Geometry: final body of the model. Coordinates: model frame, mm. Face numbers are marked on the shaded views. A direction names the side the tool comes from. Coordinates: 2 decimals unless noted, no trailing zeros. Loops run counter-clockwise (first coordinate to the right, second up) from the corner with the lowest first, then second, coordinate; pieces in that order, holes last. Notation, with made-up numbers: (-18.75, 42) - (35.25, 42) arc R21 ccw to (35.25, 62) - close; hole circle Ø7 at (46.25, 1.5). An arc over 180 degrees is marked (long way). Return JSON: item names as keys, results as strings.
from build123d import *

# Parameters (mm, degrees)
SKETCH_W        = 30
SKETCH_H        = 42
PAD_DEPTH       = 54
POCKET_DEPTH    = 42.001
POCKET001_DEPTH = 30.001
POCKET002_DEPTH = 42.001
POCKET003_DEPTH = 40.5
SKETCH005_W     = 12.884712
SKETCH005_H     = 5
PAD001_DEPTH    = 6
SKETCH006_W     = 8
SKETCH006_H     = 5
PAD002_DEPTH    = 5.5
SKETCH007_W     = 9
SKETCH007_H     = 5
PAD003_DEPTH    = 14
SKETCH009_R     = 1.75
POCKET004_DEPTH = 6
SKETCH010_W     = 16.115288
SKETCH010_H     = 23
PAD004_DEPTH    = 1
SKETCH011_W     = 16.658894
SKETCH011_H     = 16.071619
PAD005_DEPTH    = 1
PAD006_DEPTH    = 1
SKETCH015_R     = 1.125
POCKET005_DEPTH = 54.001
CHAMFER_SIZE    = 1.4
FILLET_R        = 0.5
SKETCH014_W     = 37.032941
SKETCH014_H     = 8.623624
POCKET006_DEPTH = 5
POCKET007_DEPTH = 47.501
FILLET001_R     = 2
FILLET002_R     = 1
FILLET003_R     = 1
FILLET004_R     = 1
FILLET005_R     = 1


with BuildPart() as part:
    # Sketch → Pad (new body)
    with BuildSketch(Plane.XY):
        with Locations((-28, -29)):
            Rectangle(SKETCH_W, SKETCH_H)
    extrude(amount=-PAD_DEPTH)

    # Sketch001 (on Face3 of Pad) → Pocket (cut, through all)
    with BuildSketch(Plane.XZ.offset(50)):
        with BuildLine():
            ThreePointArc((-43, -17.3161363132), (-32.0308923047, -38.9545248813), (-13, -54))
            Line((-13, -54), (-82.3272746231, -71.6955218441))
            Line((-82.3272746231, -71.6955218441), (-43, -17.3161363132))
        make_face()
    extrude(amount=-POCKET_DEPTH, mode=Mode.SUBTRACT)

    # Sketch002 (on Face3 of Pocket) → Pocket001 (cut, through all)
    with BuildSketch(Plane.YZ.offset(-13)):
        Polygon((0, 10), (-23, -65), (20.1488759761, -57.2462846327), align=None)
    extrude(amount=-POCKET001_DEPTH, mode=Mode.SUBTRACT)

    # Sketch004 (on Face6 of Pocket001) → Pocket002 (cut, through all)
    with BuildSketch(Plane.XZ.offset(50)):
        with BuildLine():
            ThreePointArc((-26, 0), (-13.3232341465, -48.8680892812), (21.51, -85.4117117262))
            Line((21.51, -85.4117117262), (74.53, 0))
            Line((-26, 0), (74.53, 0))
        make_face()
    extrude(amount=-POCKET002_DEPTH, mode=Mode.SUBTRACT)

    # Sketch003 (on Face1 of Pocket002) → Pocket003 (cut)
    with BuildSketch(Plane(origin=(0, -8, 0), x_dir=(-1, 0, 0), z_dir=(0, 1, 0))):
        with BuildLine():
            Line((42, 3), (42, -15))
            ThreePointArc((12.43, -53.2689919013), (31.9114915655, -37.7634197527), (42, -15))
            Line((12.43, -52.0274321222), (12.43, -53.2689919013))
            ThreePointArc((12.43, -52.0274321222), (23.2887545115, -27.0145266164), (27, 0))
            Line((27, 3), (27, 0))
            Line((42, 3), (27, 3))
        make_face()
    extrude(amount=-POCKET003_DEPTH, mode=Mode.SUBTRACT)

    # Sketch005 (on Face1 of Pocket003) → Pad001 (join)
    with BuildSketch(Plane(origin=(0, -8, 0), x_dir=(-1, 0, 0), z_dir=(0, 1, 0))):
        with Locations((20.442356, -2.5)):
            Rectangle(SKETCH005_W, SKETCH005_H)
    extrude(amount=-PAD001_DEPTH)

    # Sketch006 (on Face12 of Pad001) → Pad002 (join)
    with BuildSketch(Plane(origin=(0, -8, 0), x_dir=(-1, 0, 0), z_dir=(0, 1, 0))):
        with Locations((18, -2.5)):
            Rectangle(SKETCH006_W, SKETCH006_H)
    extrude(amount=PAD002_DEPTH)

    # Sketch007 (on Face11 of Pad002) → Pad003 (join)
    with BuildSketch(Plane.XZ.offset(50)):
        with Locations((-22.5, -2.5)):
            Rectangle(SKETCH007_W, SKETCH007_H)
    extrude(amount=-PAD003_DEPTH)

    # Sketch009 (on Face25 of Pad003) → Pocket004 (cut)
    with BuildSketch(Plane.XY):
        with Locations((-18, -6)):
            Circle(SKETCH009_R)
        with Locations((-22, -40)):
            Circle(SKETCH009_R)
    extrude(amount=-POCKET004_DEPTH, mode=Mode.SUBTRACT)

    # Sketch010 (on Face27 of Pocket004) → Pad004 (join)
    with BuildSketch(Plane.XY):
        with Locations((-34.942356, -38.5)):
            Rectangle(SKETCH010_W, SKETCH010_H)
    extrude(amount=-PAD004_DEPTH)

    # Sketch011 (on Face49 of Pad004) → Pad005 (join)
    with BuildSketch(Plane(origin=(0, -8, 0), x_dir=(-1, 0, 0), z_dir=(0, 1, 0))):
        with Locations((33.892149, -8.0883895)):
            Rectangle(SKETCH011_W, SKETCH011_H)
    extrude(amount=-PAD005_DEPTH)

    # Sketch013 (on Face47 of Pad005) → Pad006 (join)
    with BuildSketch(Plane(origin=(0, -2.8030549236, 0.8596035099), x_dir=(-1, 0, 0), z_dir=(0, 0.9560542082, -0.2931899572))):
        with BuildLine():
            Line((42.333473, -17.6579), (25.319201, -17.6579))
            ThreePointArc((13, -54.3247056888), (20.7764339487, -36.5345215912), (25.319201, -17.6579))
            Line((13, -54.3247056888), (13, -56.3377401542))
            ThreePointArc((13, -56.3377401542), (32.3236400181, -40.5294570505), (42.333473, -17.6579))
        make_face()
    extrude(amount=-PAD006_DEPTH)

    # Sketch015 (on Face37 of Pad006) → Pocket005 (cut, through all)
    with BuildSketch(Plane.XY):
        with Locations((-22, -40)):
            Circle(SKETCH015_R)
    extrude(amount=-POCKET005_DEPTH, mode=Mode.SUBTRACT)

    # Chamfer
    chamfer_edges = [part.edges().sort_by_distance(p)[0] for p in [
        (-13, -34.138239, -51.07776),
    ]]
    chamfer(chamfer_edges, length=CHAMFER_SIZE)

    # Fillet
    fillet_edges = [part.edges().sort_by_distance(p)[0] for p in [
        (-13.705397, -33.952813, -49.868456),
    ]]
    fillet(fillet_edges, radius=FILLET_R)

    # Sketch014 → Pocket006 (cut)
    with BuildSketch(Plane.YZ.offset(-13)):
        with Locations((-34.3443045, -56.822496)):
            Rectangle(SKETCH014_W, SKETCH014_H)
    extrude(amount=-POCKET006_DEPTH, mode=Mode.SUBTRACT)

    # Sketch017 (on Face39 of Pocket006) → Pocket007 (cut, through all)
    with BuildSketch(Plane.XZ.offset(50)):
        Polygon((-11.053677, -46.02187), (-17.304024, -54.523899), (-5.308009, -55.921494), align=None)
    extrude(amount=-POCKET007_DEPTH, mode=Mode.SUBTRACT)

    # Fillet001
    fillet001_edges = [part.edges().sort_by_distance(p)[0] for p in [
        (-18, -36, -2.5),
        (-22, -2.5, -2.5),
        (-14, -2.5, -2.5),
        (-14, -14, -2.5),
        (-18, -50, -2.5),
    ]]
    fillet(fillet001_edges, radius=FILLET001_R)

    # Fillet002
    fillet002_edges = [part.edges().sort_by_distance(p)[0] for p in [
        (-33.031819, -50, -37.694402),
    ]]
    fillet(fillet002_edges, radius=FILLET002_R)

    # Fillet003
    fillet003_edges = [part.edges().sort_by_distance(p)[0] for p in [
        (-22.099555, -50, -27.73103),
    ]]
    fillet(fillet003_edges, radius=FILLET003_R)

    # Fillet004
    fillet004_edges = [part.edges().sort_by_distance(p)[0] for p in [
        (-22.999305, -48.5, -28.027565),
    ]]
    fillet(fillet004_edges, radius=FILLET004_R)

    # Fillet005
    fillet005_edges = [part.edges().sort_by_distance(p)[0] for p in [
        (-32.8795, -48.5, -36.469763),
    ]]
    fillet(fillet005_edges, radius=FILLET005_R)


solid = part.part
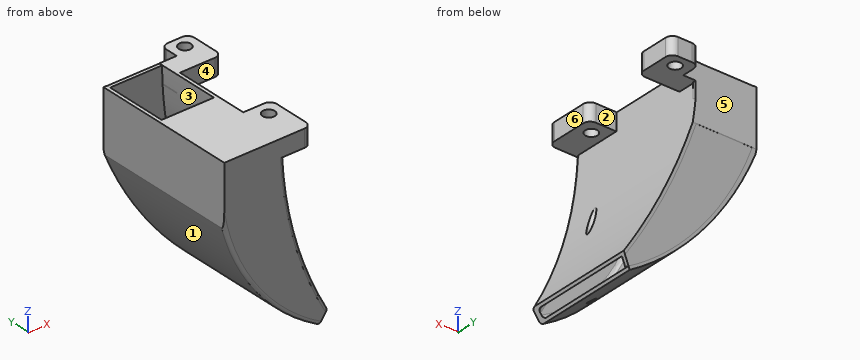
Item 1: Section query A-A, the plane y = -6. Return loops of the section in (x, z).
Worked out:
{"outline": "(-22, -5) - (-19.75, -5) - (-19.75, 0) - (-22, 0) - close; (-16.25, -5) - (-14, -5) - (-14, 0) - (-16.25, 0) - close"}
Item 2: First-contact query: pin 1 Ø3.5 at (x, y) = (-22, -40) entering from -Z; pin 2 Ø2 at (y, z) = (-39.5, -44.5) entering from +X; pin 3 Ø4 at (x, z) = (-19.5, -2.5) entering from -Y; pin 4 Ø1.5 at (y, z) = (-45, -3.5) entering from +X. Flat tips, straight axial feed; report the tip coordinate or a pass-through.
Worked out:
{"pin 1": "z = -49.78", "pin 2": "x = -15.11", "pin 3": "y = -50", "pin 4": "x = -18"}
Item 3: Ray query, probe 1 along Y at (x, z) = (-30.5, -6.5); probe 2 along Y at (x, z) = (-22, -31) (3 decimals); probe 3 along Z at (x, y) = (-38, -45). Return the intervals inside material, ascending. Write a range as from..to.
Worked out:
{"probe 1": "-50..-48.5, -9..-8", "probe 2": "-49.99..-41.125, -38.875..-12.573", "probe 3": "-30.05..-27.73, -1..0"}
Item 4: Section query C-C, the plane y = -35. Return loops of the section in (x, z) (3 decimals).
Worked out:
{"outline": "(-43, -17.316) arc R56.512 ccw to (-15.853, -52.511) - (-15.824, -52.511) - (-15.322, -51.827) arc R52.227 cw to (-42, -15) - (-42, -1) - (-26.995, -1) arc R100.176 ccw to (-13.898, -49.532) arc R0.5 ccw to (-13.752, -49.693) - (-13.247, -49.005) arc R100.53 cw to (-26, 0) - (-43, 0) - close"}
Item 5: Section query B-B, the plane y = -40. Return loops of the section in (x, z) (3 decimals), and give its area (3 significant figures).
Worked out:
{"outline": "(-43, -17.316) arc R56.512 ccw to (-23.125, -47.674) - (-23.125, -46.681) arc R52.227 cw to (-42, -15) - (-42, -1) - (-27, -1) - (-27, -5) - (-26.875, -5) arc R100.176 ccw to (-23.125, -27.593) - (-23.125, -23.87) arc R100.53 cw to (-25.876, -5) - (-23.75, -5) - (-23.75, 0) - (-43, 0) - close; (-20.875, -49.347) arc R56.512 ccw to (-15.853, -52.511) - (-15.824, -52.511) - (-15.322, -51.827) arc R52.227 cw to (-20.875, -48.376) - close; (-20.875, -34.491) arc R100.176 ccw to (-13.898, -49.532) arc R0.5 ccw to (-13.752, -49.693) - (-13.247, -49.005) arc R100.53 cw to (-20.875, -31.689) - close; (-20.25, -5) - (-18, -5) - (-18, 0) - (-20.25, 0) - close", "area": "137 mm^2"}
Item 6: Mould query, pull axis Y, two halves, no side actions, for the marked faces 4, 5 and 6. Classes: +Y half, -Y half, draft (parallel to the pull), parting line (faces both ways), or undercut.
Worked out:
{"face 4": "undercut", "face 5": "+Y half", "face 6": "draft"}
Item 7: Reachability of the marked faces 1, 2 and 3 from +Z, -Z, +X, -X, +Y, -Y: full face, straight path, thin tool, end or side. Return the list, or none.
Worked out:
{"face 1": "-Z, -X, +Y, -Y", "face 2": "+Z, +X", "face 3": "none"}
